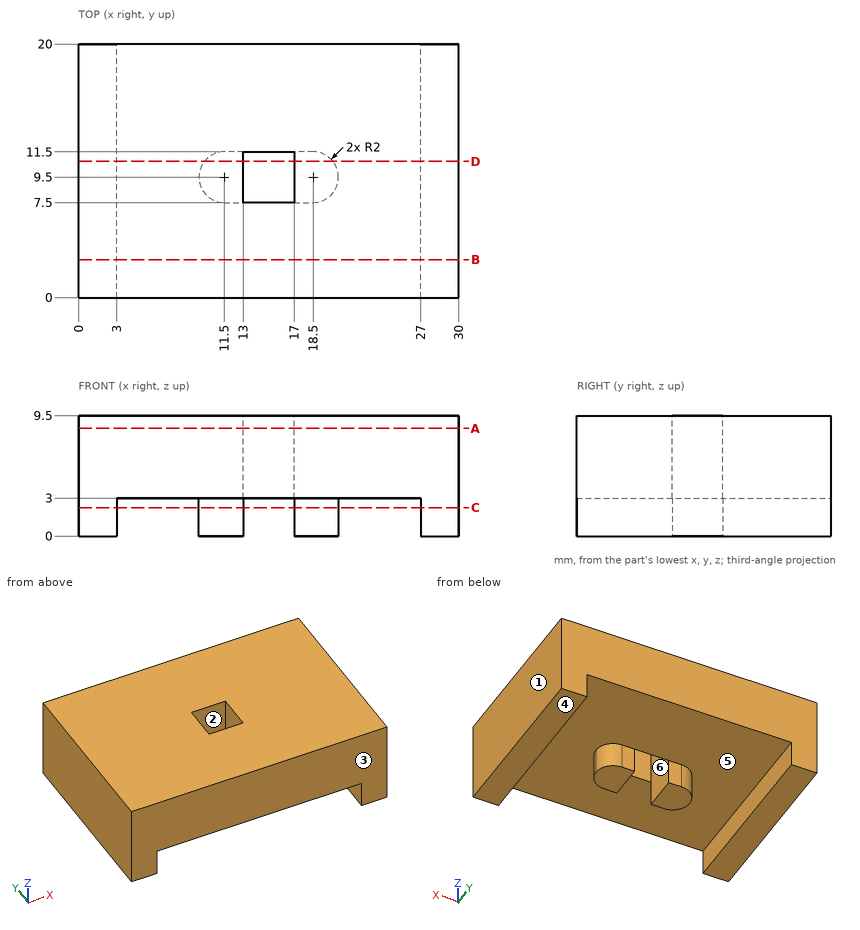
Source: three-view drawing plus pictorial views. Frame: mm from the lowest corner of the part. A direction names the side the tool comes from. Round coordinates to 2 decimals unless told otherwise and drop trailing zeros. Loops run counter-clockwise (first coordinate to the right, second up) from the corner with the lowest first, then second, coordinate; pieces in that order, holes last.
1. Access query for the marked faces 4, 5 and 6. Directions: +Z, -Z, +X, -X, +Y, -Y. A direction counts if a zero-diameter tool reaches every point of the face in a straight line with its end or side. Return the directions, or none.
2. Contact query for flat-ended pins moving along their axis: pin 1 (1.5 mm diameter, centred on x = 22.5, y = 16.5, fed in from -Z); pin 2 (0.8 mm diameter, centred on x = 12.5, z = 1.5, fed in from +Y); pin 3 (1.2 mm diameter, centred on x = 12, z = 1, fed in from -Y). Output: stop coordinate, or through.
3. Section query A-A on z = 8.5. Output: boundary loops of the cut face in (x, y).
4. Section query C-C on z = 2.25. Output: boundary loops of the cut face in (x, y), and give its area (3 significant figures).
5. Section query D-D on y = 10.75. Output: boundary loops of the cut face in (x, z).
6. Mould query, pull axis Y, two halves, no side actions, for the marked faces 1, 2 and 3. Classes: released by +Y, released by -Y, zero draft, split by the parting line, or undercut.
7. Section query B-B on y = 3. Output: boundary loops of the cut face in (x, z), and give its area (3 significant figures).
8. Ray query, L1, parallel to Y at x = 16.75, z = 6; L2, parallel to Z at x = 8, y = 1; L3, parallel to X at y = 10, z = 7.5. Return the intervals inside material, ascending.
Answers below:
1. face 4: -Z, +X, -X, +Y, -Y
1. face 5: -Z
1. face 6: +Z, -Z
2. pin 1: stops at z = 3
2. pin 2: stops at y = 11.5
2. pin 3: stops at y = 7.5
3. outline: (0, 0) - (30, 0) - (30, 20) - (0, 20) - close; hole (13, 7.5) - (17, 7.5) - (17, 11.5) - (13, 11.5) - close
4. outline: (0, 0) - (3, 0) - (3, 20) - (0, 20) - close; (11.5, 7.5) - (13, 7.5) - (13, 11.5) - (11.5, 11.5) arc R2 ccw to start; (17, 7.5) - (18.5, 7.5) arc R2 ccw to (18.5, 11.5) - (17, 11.5) - close; (27, 0) - (30, 0) - (30, 20) - (27, 20) - close
4. area: 145 mm2
5. outline: (0, 0) - (3, 0) - (3, 3) - (9.94, 3) - (9.94, 0) - (13, 0) - (13, 9.5) - (0, 9.5) - close; (17, 0) - (20.06, 0) - (20.06, 3) - (27, 3) - (27, 0) - (30, 0) - (30, 9.5) - (17, 9.5) - close
6. face 1: zero draft
6. face 2: undercut
6. face 3: released by -Y
7. outline: (0, 0) - (3, 0) - (3, 3) - (27, 3) - (27, 0) - (30, 0) - (30, 9.5) - (0, 9.5) - close
7. area: 213 mm2
8. L1: y = 0 to 7.5, 11.5 to 20
8. L2: z = 3 to 9.5
8. L3: x = 0 to 13, 17 to 30
